from build123d import *

# Parameters (mm, degrees)
SKETCH1_R               = 4
SKETCH1_R_2             = 1.5
BOSS_EXTRUDE1_DEPTH     = 6
SKETCH2_R               = 1.5000000000000004
BOSS_EXTRUDE2_DEPTH     = 1.5
CUT_EXTRUDE1_DEPTH      = 36.245567097154215
CUT_EXTRUDE1_DEPTH_BACK = 36.245567097154215
SKETCH3_R               = 1.0000000000000002
CHAMFER1_SIZE           = 0.2
FILLET1_R               = 0.2


with BuildPart() as part:
    # Sketch1 → Boss-Extrude1 (new body)
    with BuildSketch(Plane.XY):
        Circle(SKETCH1_R)
        Circle(SKETCH1_R_2, mode=Mode.SUBTRACT)
    extrude(amount=BOSS_EXTRUDE1_DEPTH)

    # Sketch2 → Boss-Extrude2 (add)
    with BuildSketch(Plane.XY):
        with BuildLine():
            Line((-3.995603052106154, 0.18750000000000017), (-2.4972519075663464, 32.1171875))
            ThreePointArc((-2.4972519075663464, 32.1171875), (1.5e-16, 34.5), (2.4972519075663464, 32.1171875))
            Line((2.4972519075663464, 32.1171875), (3.995603052106154, 0.18750000000000017))
            ThreePointArc((3.995603052106154, 0.18750000000000017), (2.4e-16, 4.000000000000002), (-3.995603052106154, 0.18750000000000017))
        make_face()
        with Locations((0, 32)):
            Circle(SKETCH2_R, mode=Mode.SUBTRACT)
    extrude(amount=BOSS_EXTRUDE2_DEPTH)

    # Sketch3 → Cut-Extrude1 (cut, two sides: drawn at the far end of the back side and taken through both)
    with BuildSketch(Plane(origin=(0, 0, 0), x_dir=(0, 0, -1), z_dir=(1, 0, 0)).offset(-CUT_EXTRUDE1_DEPTH_BACK)):
        with Locations((-3.5, 0)):
            Circle(SKETCH3_R)
    extrude(amount=CUT_EXTRUDE1_DEPTH + CUT_EXTRUDE1_DEPTH_BACK, mode=Mode.SUBTRACT)

    # Chamfer1
    # the kernel refuses this chamfer: 0.2 mm, written as the material it takes off along each edge
    with BuildSketch(Plane(origin=(0, 0, 0), x_dir=(-0.9989007630265381, 0.04687500000000028, 0), z_dir=(0.04687500000000028, 0.9989007630265381, 0))) as chamfer1_piece_1:
        Polygon((4, CHAMFER1_SIZE), (4 - CHAMFER1_SIZE, 0), (4, 0), align=None)
    revolve(axis=Axis((0, 0, 0), (0, 0, 1)), revolution_arc=182.68672418569162, mode=Mode.SUBTRACT)
    with BuildSketch(Plane(origin=(2.4972519075663464, 32.1171875, 1.5), x_dir=(0.027465652126399, 0.0012888692161212708, -0.9996219169112966), z_dir=(0.04687500000000002, -0.9989007630265381, 0))) as chamfer1_piece_2_section:
        Polygon((CHAMFER1_SIZE * 0.999621916911, -CHAMFER1_SIZE * 0.0274958766106), (-CHAMFER1_SIZE * 0.0274958766106, -CHAMFER1_SIZE * 0.999621916911), (0, 0), align=None)
    chamfer1_piece_2 = extrude(amount=32.4791610144424, mode=Mode.PRIVATE)
    chamfer1_piece_2 = chamfer1_piece_2 - Plane(origin=(0, 0, 1.4336940433446623), x_dir=(1, 0, 0), z_dir=(0, 0, -1)) * Cylinder(4, 66, mode=Mode.PRIVATE)
    add(chamfer1_piece_2, mode=Mode.SUBTRACT)
    with BuildSketch(Plane(origin=(1.1e-16, 32, 1.5), x_dir=(-0.9989007630265381, 0.04687499999999997, 0), z_dir=(-0.04687499999999997, -0.9989007630265381, 0))) as chamfer1_piece_3:
        Polygon((2.5000000000000013 - CHAMFER1_SIZE, 0), (2.5000000000000013, CHAMFER1_SIZE), (2.5000000000000013, 0), align=None)
    revolve(axis=Axis((1.1e-16, 32, 1.5), (0, 0, -1)), revolution_arc=174.62655162861682, mode=Mode.SUBTRACT)
    with BuildSketch(Plane(origin=(-4.019712580118334, -0.32627121978830154, 1.5), x_dir=(0.9985230955407449, -0.046857277355217046, 0.027495876610586282), z_dir=(0.04687500000000002, 0.9989007630265381, 0))) as chamfer1_piece_4_section:
        Polygon((CHAMFER1_SIZE * 0.999621916911, CHAMFER1_SIZE * 0.0274958766106), (-CHAMFER1_SIZE * 0.0274958766106, CHAMFER1_SIZE * 0.999621916911), (0, 0), align=None)
    chamfer1_piece_4 = extrude(amount=32.479161014442404, mode=Mode.PRIVATE)
    chamfer1_piece_4 = chamfer1_piece_4 - Plane(origin=(0, 0, 1.433694043044513), x_dir=(1, 0, 0), z_dir=(0, 0, -1)) * Cylinder(4, 66, mode=Mode.PRIVATE)
    add(chamfer1_piece_4, mode=Mode.SUBTRACT)
    with BuildSketch(Plane(origin=(0, 32, 0), x_dir=(1, 0, 0), z_dir=(0, -1, 0))) as chamfer1_piece_5:
        Polygon((1.5000000000000004 + CHAMFER1_SIZE, 0), (1.5000000000000004, CHAMFER1_SIZE), (1.5000000000000004, 0), align=None)
    revolve(axis=Axis((0, 32, 0), (0, 0, 1)), mode=Mode.SUBTRACT)
    with BuildSketch(Plane(origin=(2.4972519075663464, 32.1171875, 0), x_dir=(-0.9985230955407451, -0.04685727735521706, -0.02749587661058638), z_dir=(0.04687500000000002, -0.9989007630265381, 0))) as chamfer1_piece_6:
        Polygon((CHAMFER1_SIZE * 0.999621916911, -CHAMFER1_SIZE * 0.0274958766106), (-CHAMFER1_SIZE * 0.0274958766106, -CHAMFER1_SIZE * 0.999621916911), (0, 0), align=None)
    extrude(amount=31.96482441684922, mode=Mode.SUBTRACT)
    with BuildSketch(Plane(origin=(1.1e-16, 32, 0), x_dir=(-0.9989007630265381, 0.04687499999999997, 0), z_dir=(-0.04687499999999997, -0.9989007630265381, 0))) as chamfer1_piece_7:
        Polygon((2.5000000000000013 - CHAMFER1_SIZE, 0), (2.5000000000000013, -CHAMFER1_SIZE), (2.5000000000000013, 0), align=None)
    revolve(axis=Axis((1.1e-16, 32, 0), (0, 0, -1)), revolution_arc=174.62655162861682, mode=Mode.SUBTRACT)
    with BuildSketch(Plane(origin=(-3.995603052106154, 0.18750000000000017, 0), x_dir=(0.9985230955407449, -0.04685727735521705, -0.027495876610586376), z_dir=(0.04687500000000002, 0.9989007630265381, 0))) as chamfer1_piece_8:
        Polygon((CHAMFER1_SIZE * 0.999621916911, -CHAMFER1_SIZE * 0.0274958766106), (-CHAMFER1_SIZE * 0.0274958766106, -CHAMFER1_SIZE * 0.999621916911), (0, 0), align=None)
    extrude(amount=31.96482441684922, mode=Mode.SUBTRACT)
    with BuildSketch(Plane(origin=(0, 32, 1.5), x_dir=(1, 0, 0), z_dir=(0, -1, 0))) as chamfer1_piece_9:
        Polygon((1.5000000000000004 + CHAMFER1_SIZE, 0), (1.5000000000000004, -CHAMFER1_SIZE), (1.5000000000000004, 0), align=None)
    revolve(axis=Axis((0, 32, 1.5), (0, 0, 1)), mode=Mode.SUBTRACT)
    with BuildSketch(Plane(origin=(0, 0, 6), x_dir=(1, 0, 0), z_dir=(0, -1, 0))) as chamfer1_piece_10:
        Polygon((4, -CHAMFER1_SIZE), (4 - CHAMFER1_SIZE, 0), (4, 0), align=None)
    revolve(axis=Axis((0, 0, 6), (0, 0, 1)), mode=Mode.SUBTRACT)
    with BuildSketch(Plane(origin=(0, 0, 6), x_dir=(1, 0, 0), z_dir=(0, -1, 0))) as chamfer1_piece_11:
        Polygon((1.5 + CHAMFER1_SIZE, 0), (1.5, -CHAMFER1_SIZE), (1.5, 0), align=None)
    revolve(axis=Axis((0, 0, 6), (0, 0, 1)), mode=Mode.SUBTRACT)
    with BuildSketch(Plane(origin=(0, 0, 0), x_dir=(1, 0, 0), z_dir=(0, -1, 0))) as chamfer1_piece_12:
        Polygon((4, CHAMFER1_SIZE), (4 - CHAMFER1_SIZE, 0), (4, 0), align=None)
    revolve(axis=Axis((0, 0, 0), (0, 0, 1)), revolution_arc=2.686724185691597, mode=Mode.SUBTRACT)

    # Fillet1
    fillet1_edges = [part.edges().sort_by_distance(p)[0] for p in [
        (-1.15197e-12, 4.000000000000002, 1.5),
    ]]
    fillet(fillet1_edges, radius=FILLET1_R)


solid = part.part
Input: part model. Units: mm. Frame: model coordinates. A direction names the side the tool comes from. Give positions to 0.01 mm unless a question says otherwise; leave off trailing zeros. Order: outer loops, then holes, each group sorted by start corner. A loop starts at its lowest first (then second) coordinate and runs counter-clockwise, first axis right, second up.
Q1. Section B-B on z = 3.5. Output: boundary loops of the cut face in (x, y), and give its area (3 significant figures).
Checked values:
outline: (-3.87, -1) arc R4 ccw to (3.87, -1) - (1.12, -1) arc R1.5 cw to (-1.12, -1) - close; (-3.87, 1) - (-1.12, 1) arc R1.5 cw to (1.12, 1) - (3.87, 1) arc R4 ccw to start
area: 32.9 mm2
Q2. Ray query, probe 1 along Y at (x, z) = (0, 0.8); probe 2 along Z at (x, y) = (2.7, 0); probe 3 along Y at (x, z) = (0, 4.45). Return the intervals inside material, ascending.
Checked values:
probe 1: y = -4 to -1.5, 1.5 to 30.5, 33.5 to 34.5
probe 2: z = 0 to 2.5, 4.5 to 6
probe 3: y = -4 to -1.5, 1.5 to 4
Q3. Contact query for flat-ended pins moving along their axis: pin 1 Ø1.5 at (y, z) = (15.5, 1) entering from -X; pin 2 Ø3.5 at (x, y) = (-0.5, 14) entering from +Z; pin 3 Ø1.5 at (y, z) = (15, 1) entering from +X. Output: stop coordinate, or through.
Checked values:
pin 1: stops at x = -3.31
pin 2: stops at z = 1.5
pin 3: stops at x = 3.34
Q4. Set-up query: faces 1 (the cylindrical face through (-0.325, 30.536, 0.742)), 2 (the cylindrical face through (1.846, -3.549, 2.961)). Return all of +Z, -Z, +X, -X, +Y, -Y with unobstructed straight access to the full face (end or side cutting, diameter ignored); none if empty.
Checked values:
face 1: +Z, -Z
face 2: +Z
Q5. Draft query along Y for faces 3 (the cylindrical face through (2.539, 0.3, 2.546)), 4 (the cylindrical face through (-2.579, 0.3, 2.546)), 5 (the flat face through (0, 11, 0)), 6 (the flat face through (3.236, 16.376, 0.742)). Return one class per face: +Y half, -Y half, draft (parallel to the pull), parting line (faces both ways), or undercut.
Checked values:
face 3: undercut
face 4: undercut
face 5: draft
face 6: +Y half
Q6. Section A-A on x = 0. Output: boundary loops of the cut face in (y, z), and give its area (3 significant figures).
Checked values:
outline: (-4, 0.2) - (-3.8, 0) - (-1.5, 0) - (-1.5, 5.8) - (-1.7, 6) - (-3.8, 6) - (-4, 5.8) - close; (1.5, 0) - (30.3, 0) - (30.5, 0.2) - (30.5, 1.3) - (30.3, 1.5) - (4.2, 1.5) arc R0.2 cw to (4, 1.7) - (4, 5.8) - (3.8, 6) - (1.7, 6) - (1.5, 5.8) - close; (33.5, 0.2) - (33.7, 0) - (34.3, 0) - (34.5, 0.2) - (34.5, 1.3) - (34.3, 1.5) - (33.7, 1.5) - (33.5, 1.3) - close
area: 71.0 mm2
